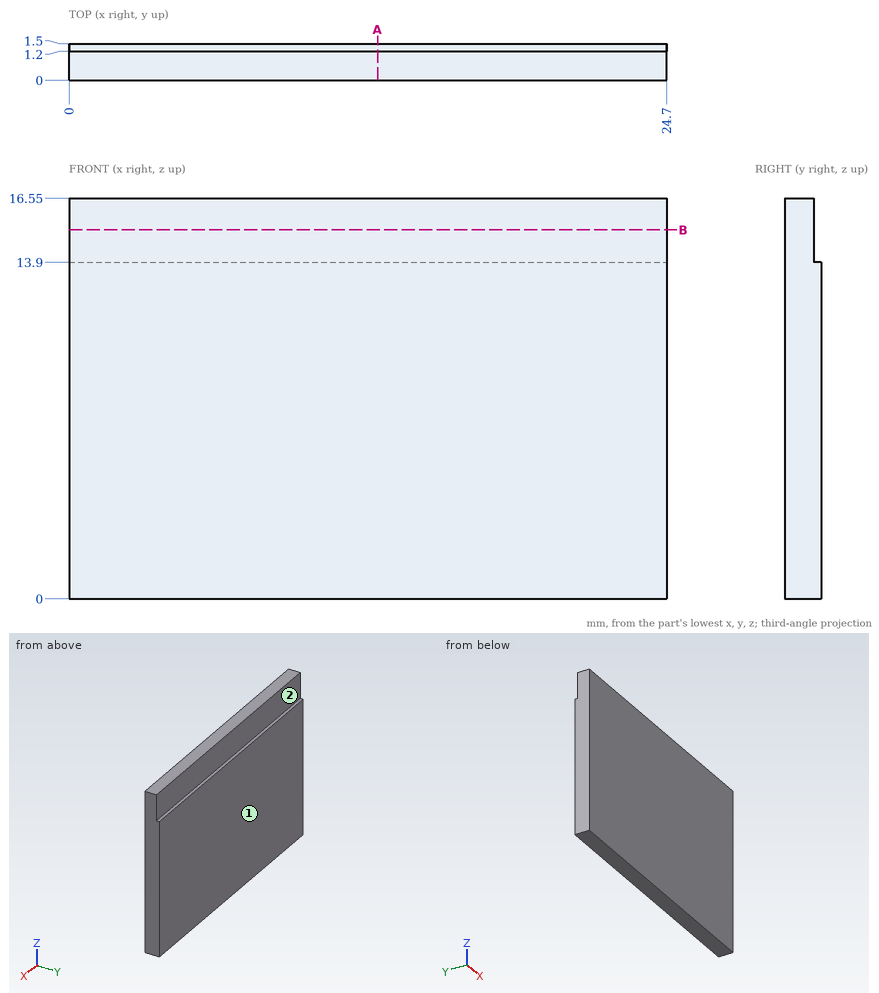
The drawing under review shows one solid part. Ordinate dimensions are in mm from its lowest x, y, z. A direction names the side the tool comes from. Round coordinates to 2 decimals unless told otherwise and drop trailing zeros. Order: outer loops, then holes, each group sorted by start corner. A loop starts at its lowest first (then second) coordinate and runs counter-clockwise, first axis right, second up. Notation, with made-up numbers: (41, -10.75) -> (57, -10.75) arc R30 ccw to (57, 19.25) -> close; hole circle Ø3 at (-9, 74). An arc over 180 degrees is marked (long way). Use a Markdown table: item, result.
Item 1: Machinability: for the marked faces 1 and 2, which of the approach directions +Z, -Z, +X, -X, +Y, -Y give a long, thin tool a straight path to every point of the face, cutting with its end or side? Answer none if there is none.
Resolved:
| item | result |
|---|---|
| face 1 | +Z, -Z, +X, -X, +Y |
| face 2 | +Z, +X, -X, +Y |
Item 2: For pin 1 (8 mm diameter, centred on x = 6, z = 13, fed in from -Y); pin 2 (0.8 mm diameter, centred on x = 13, z = 15.5, fed in from +Y), all flat-tipped, find the tip position at first contact; note any pin that passes through.
Resolved:
| item | result |
|---|---|
| pin 1 | stops at y = 0 |
| pin 2 | stops at y = 1.2 |
Item 3: Take a section at A-A (x = 12.75). State the section outline as (y, z) points.
Resolved:
| item | result |
|---|---|
| outline | (0, 0) -> (1.5, 0) -> (1.5, 13.9) -> (1.2, 13.9) -> (1.2, 16.55) -> (0, 16.55) -> close |
Item 4: For line 1 along Z through (x, y) = (19.5, 1.3); line 2 along Y through (x, z) = (7.75, 14), list the stretches that pass through material, from the lowest coordinate up. Write a range as [from, to].
Resolved:
| item | result |
|---|---|
| line 1 | z = [0, 13.9] |
| line 2 | y = [0, 1.2] |
Item 5: Take a section at B-B (z = 15.25). State the section outline as (x, y) points.
Resolved:
| item | result |
|---|---|
| outline | (0, 0) -> (24.7, 0) -> (24.7, 1.2) -> (0, 1.2) -> close |
